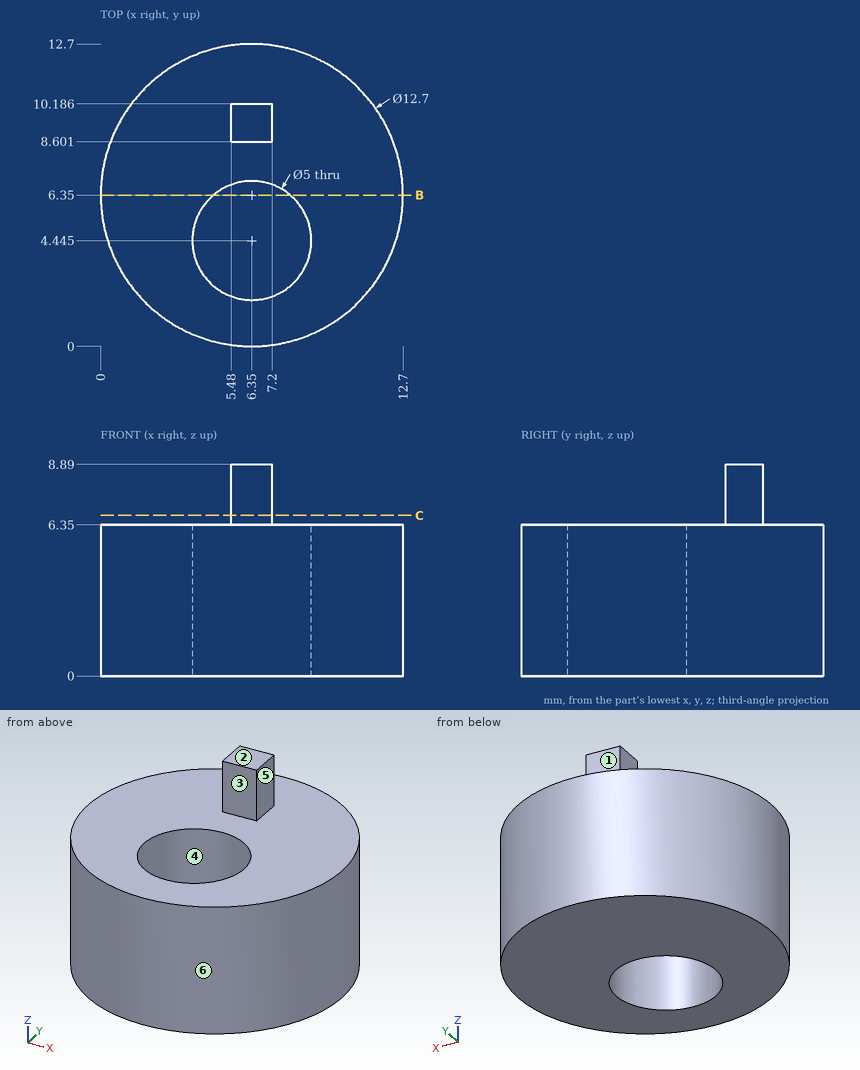
Here's the drawing with two shaded views (mm, measured from the low corner). I have some questions. A direction names the side the tool comes from. Coordinates: 2 decimals unless noted, no trailing zeros. Order: outer loops, then holes, each group sorted by start corner. A loop starts at its lowest first (then second) coordinate and runs counter-clockwise, first axis right, second up. Notation, with made-up numbers: M 44.5,86.25 L 79.5,86.25 A27 cw 79.5,117.25 Z; hole C 9.25,31.5 d6. An arc over 180 degrees is marked long. Write item = value, one per line.
(1) I need wall thicknesses on line 1 along Y through (x, z) = (6.35, 4.5) (1 decimal); line 2 along Z through (x, y) = (1.75, 7.5); line 3 along Y through (x, z) = (4.75, 6) (1 decimal). Which ranges of each line are inside material? Lowest first, please. Write a range as [from, to].
Results are:
line_1 = [0, 1.9], [6.9, 12.7]
line_2 = [0, 6.35]
line_3 = [0.2, 2.5], [6.4, 12.5]
(2) If we mould it in two halves opening along Y, with no side actions, what happens to the marked faces 1, 2, 3 and 4? For each: pulls with the +Y half, pulls with the -Y half, needs draft (parallel to the pull), parting line crosses it, or undercut.
Results are:
face_1 = pulls with the +Y half
face_2 = needs draft
face_3 = pulls with the -Y half
face_4 = undercut
(3) Suppose I cut it at B-B on y = 6.35. Please give me the cut outline in (x, z).
Results are:
outline = M 0,0 L 4.73,0 L 4.73,6.35 L 0,6.35 Z; M 7.97,0 L 12.7,0 L 12.7,6.35 L 7.97,6.35 Z
(4) Suppose I cut it at C-C on z = 6.75. Please give me the cut outline in (x, y).
Results are:
outline = M 5.48,8.6 L 7.2,8.6 L 7.2,10.19 L 5.48,10.19 Z
(5) For the marked faces 5 and 6, which set-ups out of +Z, -Z, +X, -X, +Y, -Y let a thin tool reach every point of the face, with its end or its side?
Results are:
face_5 = +Z, +X, +Y, -Y
face_6 = +Z, -Z
(6) For pin 1 Ø4 at (x, y) = (5, 5) entering from +Z; pin 2 Ø0.9 at (x, z) = (6, 7) entering from +Y; pin 3 Ø3 at (x, z) = (10.5, 3) entering from -Y, each with a flat end and sliding along its axis, tell me the tip position at first contact or that it passes through.
Results are:
pin_1 = 6.35
pin_2 = 10.19
pin_3 = 0.58
